Geometry check sheet. Reference: the model listing, model coordinates, mm. Round coordinates to 2 decimals unless told otherwise and drop trailing zeros. Order: outer loops, then holes, each group sorted by start corner. A loop starts at its lowest first (then second) coordinate and runs counter-clockwise, first axis right, second up.
(1) Cross-section at B-B on z = 0. Enter the section's corners in (x, y), and give its area (3 significant figures).
(2) Cross-section at C-C on x = 8.5. Enter the section's corners in (y, z).
(3) Gauge pin test, flat ends, axial feed: P1, Ø1.5, axis at x = 33, y = -2, coming from the -Z side; P2, Ø1.5, axis at x = 11.5, y = -1, coming from the +Z side; P3, Ø1.2, axis at y = -1, z = -3.5, coming from the -X side; P4, Ø17.5, axis at x = 0, z = 0, coming from the +Y side. Record the tip position at first contact, or that the pin passes through.
(4) Thickness scan on L1, parallel to Z at x = 48.5, y = -1.5; L2, parallel to Z at x = 20.5, y = -1.4; L3, parallel to Y at x = 47, z = 7.5. Record the ranges inside material, lowest first.
(5) Cross-section at A-A on x = 0. Enter the section's corners in (y, z), and give its area (3 significant figures).
(6) Cross-section at D-D on z = -11. Enter the section's corners in (x, y).
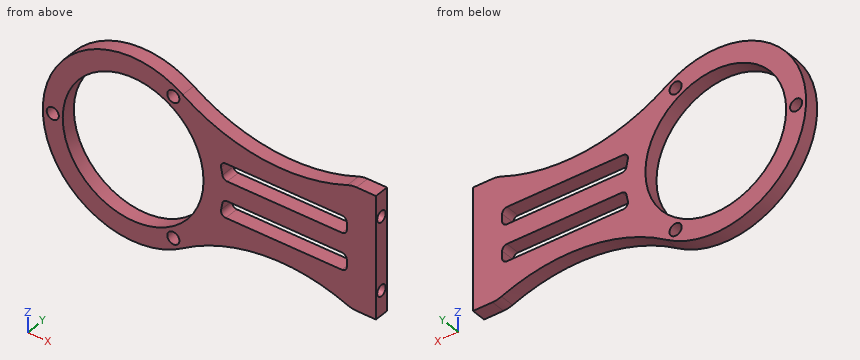
from build123d import *

# Parameters (mm, degrees)
F0_R     = 14.5
F1_DEPTH = 3
F2_D     = 2.5
F3_R     = 1
F4_R     = 5
F6_D     = 2.3
F6_DEPTH = 4
F6_TIP   = 0.6909897119


with BuildPart() as f1:
    # F0 (on Front) → F1 (new body)
    with BuildSketch(Plane.XZ):
        with BuildLine():
            ThreePointArc((18.4921605011, -2), (18.5730205583, -1.0014526146), (18.6, 0))
            ThreePointArc((18.6, 0), (18.5730205583, 1.0014526146), (18.4921605011, 2))
            ThreePointArc((18.4921605011, 2), (18.2144580261, 3.7674286742), (17.7682300751, 5.5))
            ThreePointArc((17.7682300751, 5.5), (14.8636221286, 11.1818038445), (10.2095594024, 15.5475045203))
            ThreePointArc((10.2095594024, 15.5475045203), (-18.6, 0), (10.2095594024, -15.5475045203))
            ThreePointArc((10.2095594024, -15.5475045203), (14.8636221286, -11.1818038445), (17.7682300751, -5.5))
            ThreePointArc((17.7682300751, -5.5), (18.2144580261, -3.7674286742), (18.4921605011, -2))
        make_face()
        Circle(F0_R, mode=Mode.SUBTRACT)
        with BuildLine():
            ThreePointArc((18.4921605011, 2), (18.5730205583, 1.0014526146), (18.6, 0))
            ThreePointArc((18.6, 0), (18.5730205583, -1.0014526146), (18.4921605011, -2))
            Line((18.4921605011, -2), (44, -2))
            Line((44, -2), (44, -5.5))
            Line((44, -5.5), (17.7682300751, -5.5))
            ThreePointArc((17.7682300751, -5.5), (14.8636221286, -11.1818038445), (10.2095594024, -15.5475045203))
            ThreePointArc((10.2095594024, -15.5475045203), (27.2208300421, -9.6405667001), (45, -12.5))
            Line((45, -12.5), (50, -12.5))
            Line((50, -12.5), (50, 12.5))
            Line((50, 12.5), (45, 12.5))
            ThreePointArc((45, 12.5), (27.2208300421, 9.6405667001), (10.2095594024, 15.5475045203))
            ThreePointArc((10.2095594024, 15.5475045203), (14.8636221286, 11.1818038445), (17.7682300751, 5.5))
            Line((17.7682300751, 5.5), (44, 5.5))
            Line((44, 5.5), (44, 2))
            Line((44, 2), (18.4921605011, 2))
        make_face()
    extrude(amount=F1_DEPTH)

    # F2 (through all)
    with Locations(Plane(origin=(0, 0, 0), x_dir=(1, 0, 0), z_dir=(0, 1, 0))):
        with Locations((-16.55, 0), (8.275, 14.3327204326), (8.275, -14.3327204326)):
            Hole(F2_D / 2)

    # F3
    f3_edges = [f1.edges().sort_by_distance(p)[0] for p in [
        (17.76823, -1.5, 5.5),
        (18.492161, -1.5, -2),
        (18.492161, -1.5, 2),
        (17.76823, -1.5, -5.5),
        (44, -1.5, -2),
        (44, -1.5, 5.5),
        (44, -1.5, 2),
        (44, -1.5, -5.5),
    ]]
    fillet(f3_edges, radius=F3_R)

    # F4
    f4_edges = [f1.edges().sort_by_distance(p)[0] for p in [
        (45, -1.5, 12.5),
        (45, -1.5, -12.5),
    ]]
    fillet(f4_edges, radius=F4_R)

    # F6
    with Locations(Plane.YZ.offset(50)):
        with Locations((-1.5, 7.5), (-1.5, -7.5)):
            Hole(F6_D / 2, depth=F6_DEPTH)
            with Locations((0, 0, -(F6_DEPTH + F6_TIP / 2))):  # 118° drill point
                Cone(0, F6_D / 2, F6_TIP, mode=Mode.SUBTRACT)


solid = f1.part
Found:
1. outline: (-18.6, -3) - (-17.8, -3) - (-17.8, 0) - (-18.6, 0) - close; (-15.3, -3) - (-14.5, -3) - (-14.5, 0) - (-15.3, 0) - close; (14.5, -3) - (50, -3) - (50, 0) - (14.5, 0) - close
1. area: 111 mm2
2. outline: (-3, -16.54) - (0, -16.54) - (0, -15.56) - (-3, -15.56) - close; (-3, -13.1) - (0, -13.1) - (0, -11.75) - (-3, -11.75) - close; (-3, 11.75) - (0, 11.75) - (0, 13.1) - (-3, 13.1) - close; (-3, 15.56) - (0, 15.56) - (0, 16.54) - (-3, 16.54) - close
3. P1: stops at z = -9.65
3. P2: stops at z = 15.2
3. P3: stops at x = -18.37
3. P4: passes through
4. L1: z = -12.5 to -8.65, -6.35 to 6.35, 8.65 to 12.5
4. L2: z = -10.86 to -5.5, -2 to 2, 5.5 to 10.86
4. L3: y = -3 to -2.65, -0.35 to 0
5. outline: (-3, -18.6) - (0, -18.6) - (0, -14.5) - (-3, -14.5) - close; (-3, 14.5) - (0, 14.5) - (0, 18.6) - (-3, 18.6) - close
5. area: 24.6 mm2
6. outline: (-15, -3) - (-9.45, -3) - (-9.45, 0) - (-15, 0) - close; (9.45, -3) - (20.03, -3) - (20.03, 0) - (9.45, 0) - close; (40.84, -3) - (50, -3) - (50, 0) - (40.84, 0) - close
